The model under review builds one solid part; all positions refer to its coordinate system, in mm. Face numbers are marked on the shaded views. A direction names the side the tool comes from. Give positions to 0.01 mm unless a question says otherwise; leave off trailing zeros. Order: outer loops, then holes, each group sorted by start corner. A loop starts at its lowest first (then second) coordinate and runs counter-clockwise, first axis right, second up. Notation, with made-up numbers: (22, 19.25) -> (27, 19.25) arc R27 cw to (27, 40.25) -> close; hole circle Ø5 at (27, -8.5). An arc over 180 degrees is marked (long way). Use one line per item in the form item = value.
```python
from build123d import *

# Parameters (mm, degrees)
BOSS_EXTRUDE1_DEPTH    = 10
SKETCH2_R              = 3.5
BOSS_EXTRUDE2_DEPTH    = 7.5
SKETCH3_W              = 3.66759605
SKETCH3_H              = 3.66756905
CUT_EXTRUDE1_DEPTH     = 5
BOSS_EXTRUDE3_REACH    = 20.187
CUT_EXTRUDE4_OUTLINE_W = 1.75
CUT_EXTRUDE4_OUTLINE_H = 10


# Read off the part's stored shape, not the designer's step: Cut-Extrude4
with BuildPart() as part:
    # Sketch1 → Boss-Extrude1 (new body)
    with BuildSketch(Plane.XY):
        with BuildLine():
            ThreePointArc((-2.449489743, 2.5), (0, -3.5), (2.449489743, 2.5))
            ThreePointArc((2.449489743, 2.5), (0, 3.5), (-2.449489743, 2.5))
        make_face()
        with BuildLine():
            Line((-2, 1.5), (2, 1.5))
            ThreePointArc((2, 1.5), (0, -2.5), (-2, 1.5))
        make_face(mode=Mode.SUBTRACT)
    extrude(amount=BOSS_EXTRUDE1_DEPTH)

    # Sketch2 → Boss-Extrude2 (add)
    with BuildSketch(Plane.XY.offset(10)):
        Circle(SKETCH2_R)
    extrude(amount=BOSS_EXTRUDE2_DEPTH)

    # Sketch3 → Cut-Extrude1 (cut)
    with BuildSketch(Plane.XY.offset(17.5)):
        Rectangle(SKETCH3_W, SKETCH3_H)
    extrude(amount=-CUT_EXTRUDE1_DEPTH, mode=Mode.SUBTRACT)

    # Sketch1<2> → Boss-Extrude3 (add, up to next)
    with BuildSketch(Plane.XY, mode=Mode.PRIVATE) as boss_extrude3_sk1:
        with BuildLine():
            Line((-2, 1.5), (2, 1.5))
            ThreePointArc((2, 1.5), (0, -2.5), (-2, 1.5))
        make_face()
    boss_extrude3_tool1 = extrude(boss_extrude3_sk1.sketch, amount=BOSS_EXTRUDE3_REACH, mode=Mode.PRIVATE) - part.part
    add(boss_extrude3_tool1.solids().sort_by_distance((0, -0.316718, 0))[0])

    # Cut-Extrude4 outline → Cut-Extrude4 (revolve, cut)
    with BuildSketch(Plane.XZ):
        with Locations((2.625, 5)):
            Rectangle(CUT_EXTRUDE4_OUTLINE_W, CUT_EXTRUDE4_OUTLINE_H)
    revolve(axis=Axis((0, 0, 0), (0, 0, 1)), mode=Mode.SUBTRACT)

    # Sketch6 → Revolve1 (revolve)
    with BuildSketch(Plane(origin=(0, 0, 0), x_dir=(1, 0, 0), z_dir=(0, 1, 0))):
        Polygon((-3.5, -10), (-1.75, -10), (-1.75, -8.25), align=None)
    revolve(axis=Axis((0, 0, 10), (0, 0, -1)))


solid = part.part
```
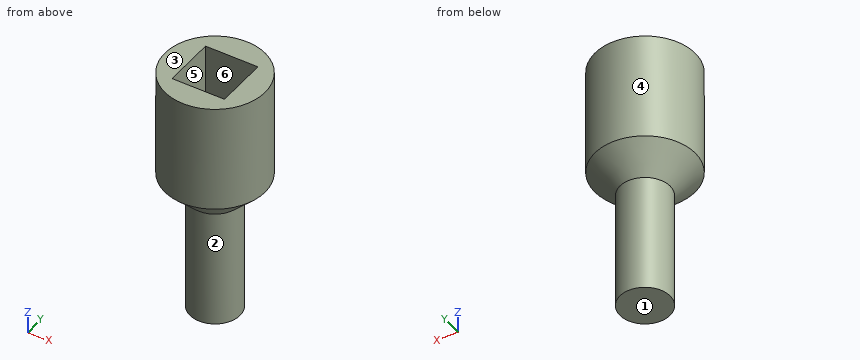
1. Tool access review of the marked faces 1 and 2: name each direction out of +Z, -Z, +X, -X, +Y, -Y from which nothing blocks a thin tool from reaching the whole face with its end or side.
Values:
face_1 = -Z, +X, -X, +Y, -Y
face_2 = -Z
2. For pin 1 Ø3 at (y, z) = (2, 13.5) entering from -X; pin 2 Ø2 at (y, z) = (-2.5, 12.5) entering from +X, all flat-tipped, find the tip position at first contact; note any pin that passes through.
Values:
pin_1 = -3.46
pin_2 = 3.16
3. Add section A-A on y = 0. Give the boundary of the cut face in (x, z).
Values:
outline = (-3.5, 10) -> (-1.75, 8.25) -> (-1.75, 0) -> (1.75, 0) -> (1.75, 8.25) -> (3.5, 10) -> (3.5, 17.5) -> (1.83, 17.5) -> (1.83, 12.5) -> (-1.83, 12.5) -> (-1.83, 17.5) -> (-3.5, 17.5) -> close
4. The part is to be moulded in two halves that separate along X. For the marked faces 3, 4, 5 and 6, say which applies: +X half, -X half, draft (parallel to the pull), parting line (faces both ways), or undercut.
Values:
face_3 = draft
face_4 = parting line
face_5 = undercut
face_6 = undercut
5. For L1, parallel to Y at x = 0.25, z = 13; L2, parallel to Y at x = -1.25, z = 14; L3, parallel to X at y = 0, z = 1.25, list the stretches that pass through material, from the lowest coordinate up.
Values:
L1 = -3.49 to -1.83, 1.83 to 3.49
L2 = -3.27 to -1.83, 1.83 to 3.27
L3 = -1.75 to 1.75
6. Add section C-C on z = 3. Give the boundary of the cut face in (x, y).
Values:
outline = circle Ø3.5 at (0, 0)
